Read the model definition and answer for the solid it produces. Units are mm, in the model's axes. Face numbers are marked on the shaded views. A direction names the side the tool comes from. Coordinates: 2 decimals unless noted, no trailing zeros. Write each loop counter-clockwise with the first axis right and the second up, starting at its lowest first coordinate (ties: lowest second). Pieces come first, ordered by that corner, then holes.
1) Each of these flat-tipped pins is pushed along its axis until it touches: pin 1 Ø5 at (x, y) = (-3, 13) entering from +Z; pin 2 Ø3 at (x, y) = (0.5, 4) entering from -Z; pin 3 Ø3 at (y, z) = (19, 0) entering from +X. Where does it stop, or does it pass through?
2) The part is cut by section B-B (x = 2.5). Determine the outline of the cut face in (y, z).
3) Which of the six approach directions +Z, -Z, +X, -X, +Y, -Y give full straight-line access (tool end or side, diameter ignored) to the marked faces 1, 2 and 3?
4) Determine the mould class of the marked faces 4, 5, 6 and 7 for opening direction Z: +Z half, -Z half, draft (parallel to the pull), parting line (faces both ways), or undercut.
5) The part is cut by section A-A (z = 0). Determine the outline of the cut face in (x, y).
6) The part is cut by section D-D (y = 9.25). Determine the outline of the cut face in (x, z).
7) Find the intervals of material crossed by line 1 (Y direction, x = 13.5, z = 0); line 2 (X direction, y = 14.5, z = 0); line 3 (Y direction, x = 3.75, z = 0), in increasing order.
8) The part is cut by section C-C (y = 19). Determine the outline of the cut face in (x, z).
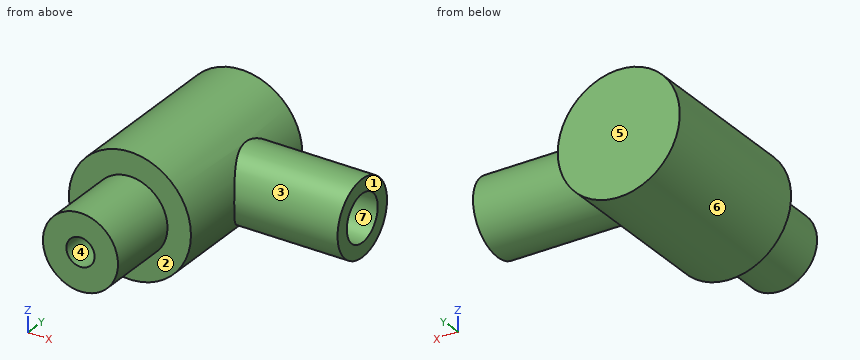
Autodesk Inventor part; units mm, degrees
ref_plane "Work Plane1" through (17.5, 0, 0) normal (1, 0, 0) x (0, 1, 0)
ref_plane "XZ Plane" through (0, 0, 0) normal (0, 1, 0) x (-1, 0, 0)
ref_plane "XY Plane" through (0, 0, 0) normal (0, 0, 1) x (1, 0, 0)
sketch "Sketch1" plane through (0, 0, 0) normal (0, 0, 1) x (1, 0, 0)
  line L0 (0, 0) -> (0, 26)
  line L1 (0, 26) -> (6.5, 26)
  line L2 (6.5, 26) -> (6.5, 8)
  line L3 (6.5, 8) -> (4, 8)
  line L4 (4, 8) -> (4, 0)
  line L5 (4, 0) -> (0, 0)
  dimension "d0" = 13
  dimension "d1" = 8
  dimension "d2" = 8
  dimension "d3" = 18
revolve "Revolution1" add sketch "Sketch1" angle 360 about axis through (0, 0, 0) along (0, 1, 0)
thread "Thread1"
ref_plane "Work Plane1" through (17.5, 0, 0) normal (1, 0, 0) x (0, 1, 0)
sketch "Sketch2" plane through (17.5, 0, 0) normal (1, 0, 0) x (0, 1, 0)
  line L0 (26, -6.5) -> (26, 6.5)
  line L1 (8, 6.5) -> (26, 6.5)
  line L2 (8, -6.5) -> (26, -6.5)
  line L3 (8, -6.5) -> (8, 6.5)
  circle A0 centre (19, 0) radius 4
  point P0 (0, 0)
  point P1 (26, 0)
  dimension "d8" = 8
  dimension "d9" = 7
extrude "Extrusion1" add sketch "Sketch2" against normal up to surface contours A0
sketch "Sketch3" plane through (17.5, 19, 0) normal (1, 0, 0) x (0, 0, -1)
  circle A0 centre (0, 0) radius 4
  point P0 (0, -19)
hole "Hole1" at (17.5, 19, 0) direction (-1, 0, 0) diameter 4 depth 17.5 counterbore diameter 5 counterbore depth 10
sketch "Sketch4" plane through (0, 0, 0) normal (0, -1, 0) x (1, 0, 0)
  circle A0 centre (0, 0) radius 4
  point P0 (0, 0)
hole "Hole2" at (0, 0, 0) direction (0, 1, 0) diameter 3 depth 20
thread "Thread2"
properties part number "157" material "Iron, Cast"
Reported:
1. pin 1: stops at z = 6.48
1. pin 2: stops at z = -4
1. pin 3: stops at x = 0
2. outline: (0, -3.12) - (8, -3.12) - (8, -6) - (26, -6) - (26, 6) - (8, 6) - (8, 3.12) - (0, 3.12) - close; hole circle Ø4 at (19, 0)
3. face 1: +Z, -Z, +X, +Y, -Y
3. face 2: -Y
3. face 3: +X
4. face 4: undercut
4. face 5: draft
4. face 6: parting line
4. face 7: undercut
5. outline: (-6.5, 8) - (-4, 8) - (-4, 0) - (-1.5, 0) - (-1.5, 20) - (0, 20) - (0, 21) - (7.5, 21) - (7.5, 21.5) - (17.5, 21.5) - (17.5, 23) - (6.5, 23) - (6.5, 26) - (-6.5, 26) - close; (1.5, 0) - (4, 0) - (4, 8) - (6.5, 8) - (6.5, 15) - (17.5, 15) - (17.5, 16.5) - (7.5, 16.5) - (7.5, 17) - (1.5, 17) - close
6. outline: circle Ø13 at (0, 0); hole circle Ø3 at (0, 0)
7. line 1: y = 15 to 16.5, 21.5 to 23
7. line 2: x = -6.5 to -1.5, 1.5 to 6.5
7. line 3: y = 0 to 17, 21 to 26
8. outline: (0, -2) - (0, -1.5) arc R1.5 cw to (0, 1.5) - (0, 2) - (7.5, 2) - (7.5, 2.5) - (17.5, 2.5) - (17.5, 4) - (5.12, 4) arc R6.5 ccw (long way) to (5.12, -4) - (17.5, -4) - (17.5, -2.5) - (7.5, -2.5) - (7.5, -2) - close
